Geometry check sheet. Reference: drawing and pictorial views, mm from the part's lowest x, y, z. A direction names the side the tool comes from. Give positions to 0.01 mm unless a question says otherwise; leave off trailing zeros. Loops run counter-clockwise (first coordinate to the right, second up) from the corner with the lowest first, then second, coordinate; pieces in that order, holes last. Notation, with made-up numbers: M -29,-32.75 L 7,-32.75 A21 ccw 7,-5.75 Z; hole C 1.5,37.25 d2. An arc over 180 degrees is marked long. Put each result on its own line as item: value. Start each with the question number.
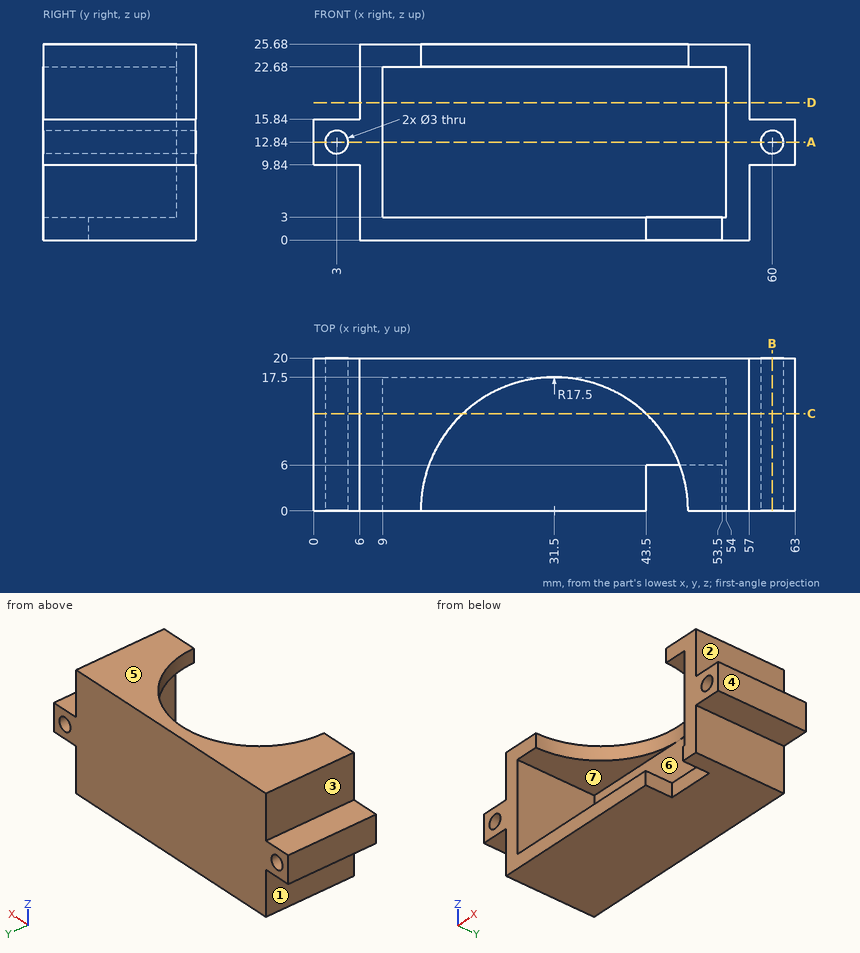
Q1. Section check C-C, the plane y = 12.75. Record the cut outline in (x, z), then the cut area to 3 significant figures.
Q2. Section check D-D, the plane z = 18. Record the cut outline in (x, y), then the cut area to 4 significant figures.
Q3. Depth check by flat-ended pin: P1, Ø9, axis at x = 17.5, y = 9.5, coming from the -Z side; P2, Ø8, axis at x = 42, z = 13.5, coming from the -Y side; P3, Ø5, axis at x = 60.5, y = 10, coming from the +Z side; P4, Ø1.5, axis at y = 2.5, z = 1.5, coming from the -X side. Enter the tip coordinate at first touch or a pass-through.
Q4. Section check B-B, the plane x = 60. Record the cut outline in (y, z).
Q5. Access from +Z, -Z, +X, -X, +Y, -Y to the whole of each face (thin tool, end or side, straight path). Record for the marked faces 1, 2 and 3.
Q6. Mould release check, pull along Z, two halves, no side actions. Record for the marked faces 4, 5, 6 and 7: pulls with the +Z half, pulls with the -Z half, needs draft (parallel to the pull), parting line crosses it, or undercut.
Q7. Section check A-A, the plane z = 12.84. Record the cut outline in (x, y), then the cut area to 4 significant figures.
Q8. Thickness scan on line 1 along X through (y, z) = (7.25, 10.75); line 2 along Z through (x, y) = (51, 10.75); line 3 along Z through (x, y) = (60, 9.5). Record the ranges inside material, lowest first. Write a range as [from, to].
Found:
1. outline: M 0,9.84 L 6,9.84 L 6,0 L 57,0 L 57,9.84 L 63,9.84 L 63,15.84 L 57,15.84 L 57,25.68 L 43.49,25.68 L 43.49,22.68 L 54,22.68 L 54,3 L 9,3 L 9,22.68 L 19.51,22.68 L 19.51,25.68 L 6,25.68 L 6,15.84 L 0,15.84 Z; hole C 3,12.84 d3; hole C 60,12.84 d3
1. area: 410 mm^2
2. outline: M 6,0 L 9,0 L 9,17.5 L 54,17.5 L 54,0 L 57,0 L 57,20 L 6,20 Z
2. area: 232.5 mm^2
3. P1: stops at z = 0
3. P2: stops at y = 17.5
3. P3: stops at z = 15.84
3. P4: stops at x = 6
4. outline: M 0,9.84 L 20,9.84 L 20,11.34 L 0,11.34 Z; M 0,14.34 L 20,14.34 L 20,15.84 L 0,15.84 Z
5. face 1: -Z, -X, +Y, -Y
5. face 2: +Z, +X, +Y, -Y
5. face 3: +Z, -X, +Y, -Y
6. face 4: needs draft
6. face 5: pulls with the +Z half
6. face 6: undercut
6. face 7: undercut
7. outline: M 0,0 L 1.5,0 L 1.5,20 L 0,20 Z; M 4.5,0 L 9,0 L 9,17.5 L 54,17.5 L 54,0 L 58.5,0 L 58.5,20 L 4.5,20 Z; M 61.5,0 L 63,0 L 63,20 L 61.5,20 Z
7. area: 352.5 mm^2
8. line 1: x = [0, 9], [54, 63]
8. line 2: z = [0, 3], [22.68, 25.68]
8. line 3: z = [9.84, 11.34], [14.34, 15.84]
